Autodesk Inventor part; units mm, degrees
ref_plane "YZ Plane" through (0, 0, 0) normal (1, 0, 0) x (0, 1, 0)
ref_plane "XZ Plane" through (0, 0, 0) normal (0, 1, 0) x (-1, 0, 0)
ref_plane "XY Plane" through (0, 0, 0) normal (0, 0, 1) x (1, 0, 0)
sketch "Sketch1" plane through (0, 0, 0) normal (0, 1, 0) x (-1, 0, 0)
  line L0 (13.46, 17) -> (-13.46, 17)
  line L1 (-16.5, 13.96) -> (-16.5, -13.96)
  line L2 (16.5, -13.96) -> (16.5, 13.96)
  line L3 (6, -19) -> (6, 9) construction
  line L4 (8.5, -17) -> (8.5, 9)
  line L5 (3.5, 9) -> (3.5, -17)
  arc A0 (8.5, 9) -> (3.5, 9) centre (6, 9) ccw
  circle A1 centre (-6.5, 10) radius 2.5
  circle A2 centre (-6.5, -10) radius 2.5
  line L6 (-13.46, -17) -> (3.5, -17)
  line L7 (8.5, -17) -> (13.46, -17)
  arc A3 (13.46, -17) -> (16.5, -13.96) centre (13.46, -13.96) ccw
  arc A4 (16.5, 13.96) -> (13.46, 17) centre (13.46, 13.96) ccw
  arc A5 (-13.46, 17) -> (-16.5, 13.96) centre (-13.46, 13.96) ccw
  arc A6 (-16.5, -13.96) -> (-13.46, -17) centre (-13.46, -13.96) ccw
  point P0 (0, 0)
  point P1 (-16.5, -17)
  point P2 (-16.5, 17)
  point P3 (16.5, -17)
  point P4 (16.5, 0)
  point P5 (0, -17)
  point P6 (6, -5)
  dimension "d0" = 33
  dimension "d1" = 34
  dimension "d2" = 5
  dimension "d4" = 28
  dimension "d5" = 8
  dimension "d6" = 5
  dimension "d7" = 5
  dimension "d8" = 20
  dimension "d9" = 10
  dimension "d10" = 7
  dimension "d11" = 3.04
extrude "Extrusion1" add sketch "Sketch1" along normal blind 12
sketch "Sketch2" plane through (-16.5, 0, -13.96) normal (-1, 0, 0) x (0, 0, 1)
  circle A0 centre (13.96, 6) radius 4
  circle A1 centre (3.96, 6) radius 2.5
  line L0 (0, 0) -> (27.92, 0)
  point P0 (13.96, 0)
  point P1 (13.96, 0)
  dimension "d14" = 8
  dimension "d15" = 5
  dimension "d16" = 6
  dimension "d17" = 10
hole "Hole1" at (-16.5, 6, 0) direction (1, 0, 0) diameter 6.647 depth 40 tip angle 118
hole "Hole2" at (-16.5, 6, -10) direction (1, 0, 0) diameter 4.134 depth 10 tip angle 118
sketch "Sketch3" plane through (0, 12, 0) normal (0, 1, 0) x (1, 0, 0)
  circle A0 centre (6.5, 10) radius 2.5
  circle A1 centre (6.5, -10) radius 2.5
  circle A2 centre (6.5, 10) radius 4.5
  circle A3 centre (6.5, -10) radius 4.5
  point P0 (0, 0)
  dimension "d32" = 9
  dimension "d33" = 9
extrude "Extrusion2" cut sketch "Sketch3" against normal blind 2
sketch "Sketch4" plane through (0, 0, 0) normal (0, -1, 0) x (1, 0, 0)
  circle A0 centre (6.5, 10) radius 2.5
  circle A1 centre (6.5, -10) radius 2.5
  line L0 (4.1906, 6) -> (1.8812, 10)
  line L1 (1.8812, 10) -> (4.1906, 14)
  line L2 (4.1906, 14) -> (8.8094, 14)
  line L3 (8.8094, 14) -> (11.1188, 10)
  line L4 (11.1188, 10) -> (8.8094, 6)
  line L5 (8.8094, 6) -> (4.1906, 6)
  line L6 (8.8094, -6) -> (11.1188, -10)
  line L7 (11.1188, -10) -> (8.8094, -14)
  line L8 (8.8094, -14) -> (4.1906, -14)
  line L9 (4.1906, -14) -> (1.8812, -10)
  line L10 (1.8812, -10) -> (4.1906, -6)
  line L11 (4.1906, -6) -> (8.8094, -6)
  point P0 (0, 0)
  dimension "d36" = 8
  dimension "d37" = 8
extrude "Extrusion3" cut sketch "Sketch4" against normal blind 5
properties part number "Anti-Backlash Nut Block" material "Aluminum 6061"
The listing builds one solid part. Answer for the finished solid, in the listing's coordinates (mm). A direction names the side the tool comes from. Round coordinates to 2 decimals unless told otherwise and drop trailing zeros. Order: outer loops, then holes, each group sorted by start corner. A loop starts at its lowest first (then second) coordinate and runs counter-clockwise, first axis right, second up. Notation, with made-up numbers: (8, 85) -> (18, 85) arc R20 ccw to (18, 121) -> close; hole circle Ø5 at (-7, 10). An arc over 180 degrees is marked (long way). Answer as CSV lines item,"result".
Q1. Consider line 1 (Y direction, x = -12.75, z = 0); line 2 (Z direction, x = 10.5, y = 6); line 3 (Z direction, x = 8, y = 7). Determine where each line is inside the solid, lowest interval first. Write a range as from..to.
Computed values:
line 1,"y = 0..2.68, 9.32..12"
line 2,"z = -17..-3.32, 3.32..17"
line 3,"z = -17..-12, -8..-3.17, 3.17..8, 12..17"
Q2. A cutting plane is placed at C-C on y = 10.5. Determine the outline of the cut face in (x, z), plus the area to 3 significant figures.
Computed values:
outline,"(-16.5, -13.96) arc R3.04 ccw to (-13.46, -17) -> (-8.5, -17) -> (-8.5, 9) arc R2.5 cw to (-3.5, 9) -> (-3.5, -17) -> (13.46, -17) arc R3.04 ccw to (16.5, -13.96) -> (16.5, 13.96) arc R3.04 ccw to (13.46, 17) -> (-13.46, 17) arc R3.04 ccw to (-16.5, 13.96) -> close; hole circle Ø9 at (6.5, -10); hole circle Ø9 at (6.5, 10)"
area,"847 mm^2"
Q3. A cutting plane is placed at B-B on x = 7. Give the number of separate pieces and of enclosed holes in the cut face, plus the area to 3 significant figures.
Computed values:
separate pieces,"3"
enclosed holes,"1"
area,"209 mm^2"
Q4. A cutting plane is placed at A-A on z = 4. Determine the outline of the cut face in (x, y).
Computed values:
outline,"(-16.5, 0) -> (-8.5, 0) -> (-8.5, 12) -> (-16.5, 12) -> close; (-3.5, 0) -> (16.5, 0) -> (16.5, 12) -> (-3.5, 12) -> close"
Q5. A cutting plane is placed at D-D on y = 6.75. Determine the outline of the cut face in (x, z).
Computed values:
outline,"(-16.5, -13.96) arc R3.04 ccw to (-13.46, -17) -> (-8.5, -17) -> (-8.5, -11.93) -> (-16.5, -11.93) -> close; (-16.5, -8.07) -> (-8.5, -8.07) -> (-8.5, -3.24) -> (-16.5, -3.24) -> close; (-16.5, 3.24) -> (-8.5, 3.24) -> (-8.5, 9) arc R2.5 cw to (-3.5, 9) -> (-3.5, 3.24) -> (16.5, 3.24) -> (16.5, 13.96) arc R3.04 ccw to (13.46, 17) -> (-13.46, 17) arc R3.04 ccw to (-16.5, 13.96) -> close; (-3.5, -17) -> (13.46, -17) arc R3.04 ccw to (16.5, -13.96) -> (16.5, -3.24) -> (-3.5, -3.24) -> close; hole circle Ø5 at (6.5, -10); hole circle Ø5 at (6.5, 10)"
Q6. Which of the six approach directions +Z, -Z, +X, -X, +Y, -Y give full straight-line access (tool end or side, diameter ignored) to faces 5 (the flat face through (9.948, 2.465, 12.028)), 6 (the flat face through (-3.5, 6, -4)), 7 (the cylindrical face through (5.91, 11.01, -14.46)), 8 (the flat face through (0, 12, 0))?
Computed values:
face 5,"-Y"
face 6,"-Z, +Y, -Y"
face 7,"+Y"
face 8,"+Z, -Z, +X, -X, +Y"
Q7. Given pin 1 (3 mm diameter, centred on x = 6.5, z = 10, fed in from +Y); pin 2 (8 mm diameter, centred on x = 6.5, z = 10, fed in from +Y); pin 3 (2.5 mm diameter, centred on x = 5, z = 11.5, fed in from -Y), each flat-ended and moving along its own axis, determine where each tip first touches the part or whether it passes through.
Computed values:
pin 1,"passes through"
pin 2,"stops at y = 10"
pin 3,"stops at y = 5"
Q8. For a pull along X with two mould halves and no side action, classify faces 1 (the cylindrical face through (6.64, 3.2, 1.79)), 2 (the cylindrical face through (5.52, 11.01, 14.39)), 3 (the cylindrical face through (-15.63, 5.92, -16.09)), 4 (the flat face through (9.98, 2.46, 8.03)) as +X half, -X half, draft (parallel to the pull), parting line (faces both ways), or undercut.
Computed values:
face 1,"draft"
face 2,"undercut"
face 3,"-X half"
face 4,"undercut"
